Model file for the job. Use its own axes, mm. Face numbers are marked on the shaded views. Coordinates: 2 decimals unless noted, no trailing zeros. Loops run counter-clockwise (first coordinate to the right, second up) from the corner with the lowest first, then second, coordinate; pieces in that order, holes last.
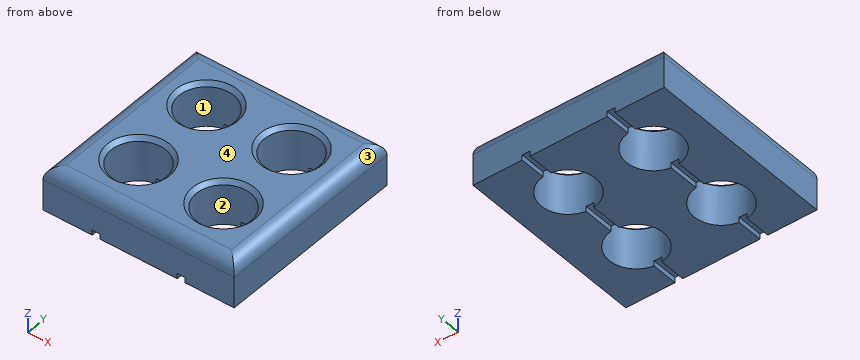
from build123d import *

# Parameters (mm, degrees)
F0_W     = 73.85
F0_H     = 73.85
F0_R     = 10.5
F1_DEPTH = 17
F2_SIZE  = 1.5
F3_R     = 5
F5_DEPTH = 2


with BuildPart() as f1:
    # F0 (on Top) → F1 (new body)
    with BuildSketch(Plane.XY):
        with Locations((16.425, -16.425)):
            Rectangle(F0_W, F0_H)
        with Locations((0, -32.85)):
            Circle(F0_R, mode=Mode.SUBTRACT)
        with Locations((32.85, -32.85)):
            Circle(F0_R, mode=Mode.SUBTRACT)
        Circle(F0_R, mode=Mode.SUBTRACT)
        with Locations((32.85, 0)):
            Circle(F0_R, mode=Mode.SUBTRACT)
    extrude(amount=F1_DEPTH)

    # F2
    f2_edges = [f1.edges().sort_by_distance(p)[0] for p in [
        (-10.5, 0, 17),
        (22.35, 0, 17),
        (22.35, -32.85, 17),
        (-10.5, -32.85, 17),
    ]]
    chamfer(f2_edges, length=F2_SIZE)

    # F3
    f3_edges = [f1.edges().sort_by_distance(p)[0] for p in [
        (16.425, -53.35, 17),
        (-20.5, -16.425, 17),
        (16.425, 20.5, 17),
        (53.35, -16.425, 17),
    ]]
    fillet(f3_edges, radius=F3_R)

    # F4 (on face) → F5 (cut)
    with BuildSketch(Plane(origin=(0, 0, 0), x_dir=(1, 0, 0), z_dir=(0, 0, -1))):
        with BuildLine():
            Line((-1.5, -10.392305), (-1.5, -20.5))
            Line((-1.5, -20.5), (1.5, -20.5))
            Line((1.5, -20.5), (1.5, -10.392305))
            ThreePointArc((1.5, -10.392305), (0, -10.5), (-1.5, -10.392305))
        make_face()
        with BuildLine():
            Line((1.5, 53.35), (-1.5, 53.35))
            Line((-1.5, 53.35), (-1.5, 43.242305))
            ThreePointArc((-1.5, 43.242305), (0, 43.35), (1.5, 43.242305))
            Line((1.5, 43.242305), (1.5, 53.35))
        make_face()
        with BuildLine():
            ThreePointArc((1.5, 43.242305), (0, 43.35), (-1.5, 43.242305))
            Line((-1.5, 43.242305), (-1.5, 22.457695))
            ThreePointArc((-1.5, 22.457695), (0, 22.35), (1.5, 22.457695))
            Line((1.5, 22.457695), (1.5, 43.242305))
        make_face()
        with BuildLine():
            ThreePointArc((1.5, 22.457695), (0, 22.35), (-1.5, 22.457695))
            Line((-1.5, 22.457695), (-1.5, 10.392305))
            ThreePointArc((-1.5, 10.392305), (0, 10.5), (1.5, 10.392305))
            Line((1.5, 10.392305), (1.5, 22.457695))
        make_face()
        with BuildLine():
            Line((34.35, 53.35), (31.35, 53.35))
            Line((31.35, 53.35), (31.35, 43.242305))
            ThreePointArc((31.35, 43.242305), (32.85, 43.35), (34.35, 43.242305))
            Line((34.35, 43.242305), (34.35, 53.35))
        make_face()
        with BuildLine():
            ThreePointArc((34.35, 22.457695), (32.85, 22.35), (31.35, 22.457695))
            Line((31.35, 22.457695), (31.35, 10.392305))
            ThreePointArc((31.35, 10.392305), (32.85, 10.5), (34.35, 10.392305))
            Line((34.35, 10.392305), (34.35, 22.457695))
        make_face()
        with BuildLine():
            ThreePointArc((34.35, 43.242305), (32.85, 43.35), (31.35, 43.242305))
            Line((31.35, 43.242305), (31.35, 22.457695))
            ThreePointArc((31.35, 22.457695), (32.85, 22.35), (34.35, 22.457695))
            Line((34.35, 22.457695), (34.35, 43.242305))
        make_face()
        with BuildLine():
            Line((31.35, -10.392305), (31.35, -20.5))
            Line((31.35, -20.5), (34.35, -20.5))
            Line((34.35, -20.5), (34.35, -10.392305))
            ThreePointArc((34.35, -10.392305), (32.85, -10.5), (31.35, -10.392305))
        make_face()
    extrude(amount=-F5_DEPTH, mode=Mode.SUBTRACT)


solid = f1.part
Q1. Mould opens along X. For the marked faces 1, 2, 3 and 4 say: +X half, -X half, draft (parallel to the pull), parting line (faces both ways), or undercut.
Answers:
face 1: undercut
face 2: undercut
face 3: +X half
face 4: draft
Q2. Slice it at A-A (y = -32.85). List the corners of the cut face in (x, z).
Answers:
outline: (-20.5, 0) - (-10.5, 0) - (-10.5, 15.5) - (-12, 17) - (-15.5, 17) arc R5 ccw to (-20.5, 12) - close; (10.5, 0) - (22.35, 0) - (22.35, 15.5) - (20.85, 17) - (12, 17) - (10.5, 15.5) - close; (43.35, 0) - (53.35, 0) - (53.35, 12) arc R5 ccw to (48.35, 17) - (44.85, 17) - (43.35, 15.5) - close
Q3. Drill centre lines: line 1 (Y direction, x = 0, z = 11.25); line 2 (X direction, y = -32.85, z = 10.75); line 3 (X direction, y = -32.85, z = 12.25). Where is each one in solid material? Low to high.
Answers:
line 1: y = -53.35 to -43.35, -22.35 to -10.5, 10.5 to 20.5
line 2: x = -20.5 to -10.5, 10.5 to 22.35, 43.35 to 53.35
line 3: x = -20.49 to -10.5, 10.5 to 22.35, 43.35 to 53.34
Q4. Flat gauge pins, fed straight in: P1, Ø5, axis at x = 26.5, z = 15, coming from the -Y side; P2, Ø0.9, axis at x = 32, y = -46, coming from the -Z side; P3, Ø10, axis at y = -11.5, z = 12.5, coming from the -X side; P4, Ø17, axis at x = 32.85, y = -32.85, coming from the -Z side. Where does each tip first touch, or does it go through?
Answers:
P1: stops at y = -53.32
P2: stops at z = 2
P3: stops at x = -20.5
P4: passes through
Q5. Slice it at C-C (z = 9.5). List the corners of the cut face in (x, y).
Answers:
outline: (-20.5, -53.35) - (53.35, -53.35) - (53.35, 20.5) - (-20.5, 20.5) - close; hole circle Ø21 at (0, -32.85); hole circle Ø21 at (0, 0); hole circle Ø21 at (32.85, -32.85); hole circle Ø21 at (32.85, 0)
Q6. Slice it at B-B (x = 0). List the corners of the cut face in (y, z).
Answers:
outline: (-53.35, 2) - (-43.35, 2) - (-43.35, 15.5) - (-44.85, 17) - (-48.35, 17) arc R5 ccw to (-53.35, 12) - close; (-22.35, 2) - (-10.5, 2) - (-10.5, 15.5) - (-12, 17) - (-20.85, 17) - (-22.35, 15.5) - close; (10.5, 2) - (20.5, 2) - (20.5, 12) arc R5 ccw to (15.5, 17) - (12, 17) - (10.5, 15.5) - close
